Drawing for the job (mm, zero at the part's lowest x, y, z). A direction names the side the tool comes from. Give positions to 0.01 mm unless a question says otherwise; leave off trailing zeros. Order: outer loops, then holes, each group sorted by start corner. A loop starts at its lowest first (then second) coordinate and runs counter-clockwise, first axis right, second up. Notation, with made-up numbers: (-34, -38) - (-8, -38) arc R9 cw to (-8, -26) - close; hole circle Ø6 at (26, 45.5). An arc over 180 degrees is marked (long way). One line per item, written item: value.
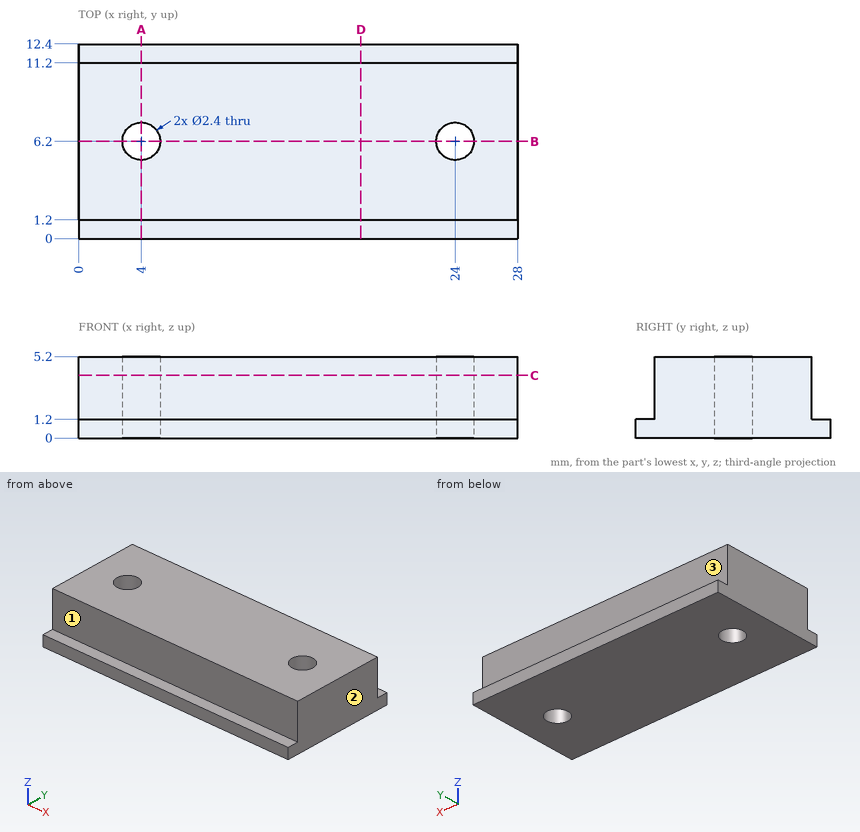
(1) Slice it at A-A, the plane x = 4. Give the cut face in (y, z).
Completed:
outline: (0, 0) - (5, 0) - (5, 5.2) - (1.2, 5.2) - (1.2, 1.2) - (0, 1.2) - close; (7.4, 0) - (12.4, 0) - (12.4, 1.2) - (11.2, 1.2) - (11.2, 5.2) - (7.4, 5.2) - close
(2) Slice it at C-C, the plane z = 4. Give the cut face in (x, y).
Completed:
outline: (0, 1.2) - (28, 1.2) - (28, 11.2) - (0, 11.2) - close; hole circle Ø2.4 at (4, 6.2); hole circle Ø2.4 at (24, 6.2)
(3) Slice it at B-B, the plane y = 6.2. Give the cut face in (x, z), and give its area (3 significant figures).
Completed:
outline: (0, 0) - (2.8, 0) - (2.8, 5.2) - (0, 5.2) - close; (5.2, 0) - (22.8, 0) - (22.8, 5.2) - (5.2, 5.2) - close; (25.2, 0) - (28, 0) - (28, 5.2) - (25.2, 5.2) - close
area: 121 mm²
(4) Pin check, flat tips, straight feed: P1, Ø0.6, axis at x = 11.5, y = 0.5, coming from the +Z side; P2, Ø3, axis at x = 14, z = 3.5, coming from the -Y side; P3, Ø2, axis at x = 12.5, z = 3.5, coming from the +Y side. Stop position of each tip, or through.
Completed:
P1: z = 1.2
P2: y = 1.2
P3: y = 11.2
(5) 3-axis set-ups, long thin cutter, end or side, ignore diameter. For the marked faces 1, 2 and 3: which of +Z, -Z, +X, -X, +Y, -Y reach the whole face in a straight line?
Completed:
face 1: +Z, +X, -X, -Y
face 2: +Z, -Z, +X, +Y, -Y
face 3: +Z, +X, -X, +Y
(6) Drill centre lines: line 1 (Y direction, x = 4, z = 1.95); line 2 (X direction, y = 6.75, z = 4.3); line 3 (Y direction, x = 10, z = 3.2). Where is each one in solid material? Low to high.
Completed:
line 1: 1.2 to 5, 7.4 to 11.2
line 2: 0 to 2.93, 5.07 to 22.93, 25.07 to 28
line 3: 1.2 to 11.2
(7) Slice it at D-D, the plane x = 18. Give the cut face in (y, z).
Completed:
outline: (0, 0) - (12.4, 0) - (12.4, 1.2) - (11.2, 1.2) - (11.2, 5.2) - (1.2, 5.2) - (1.2, 1.2) - (0, 1.2) - close
